Answer from the drawing. Dimensions are ordinates in mm from the lowest x, y and z of the part. A direction names the side the tool comes from. Coordinates: 2 decimals unless noted, no trailing zeros. Loops run counter-clockwise (first coordinate to the right, second up) from the corner with the lowest first, then second, coordinate; pieces in that order, holes last.
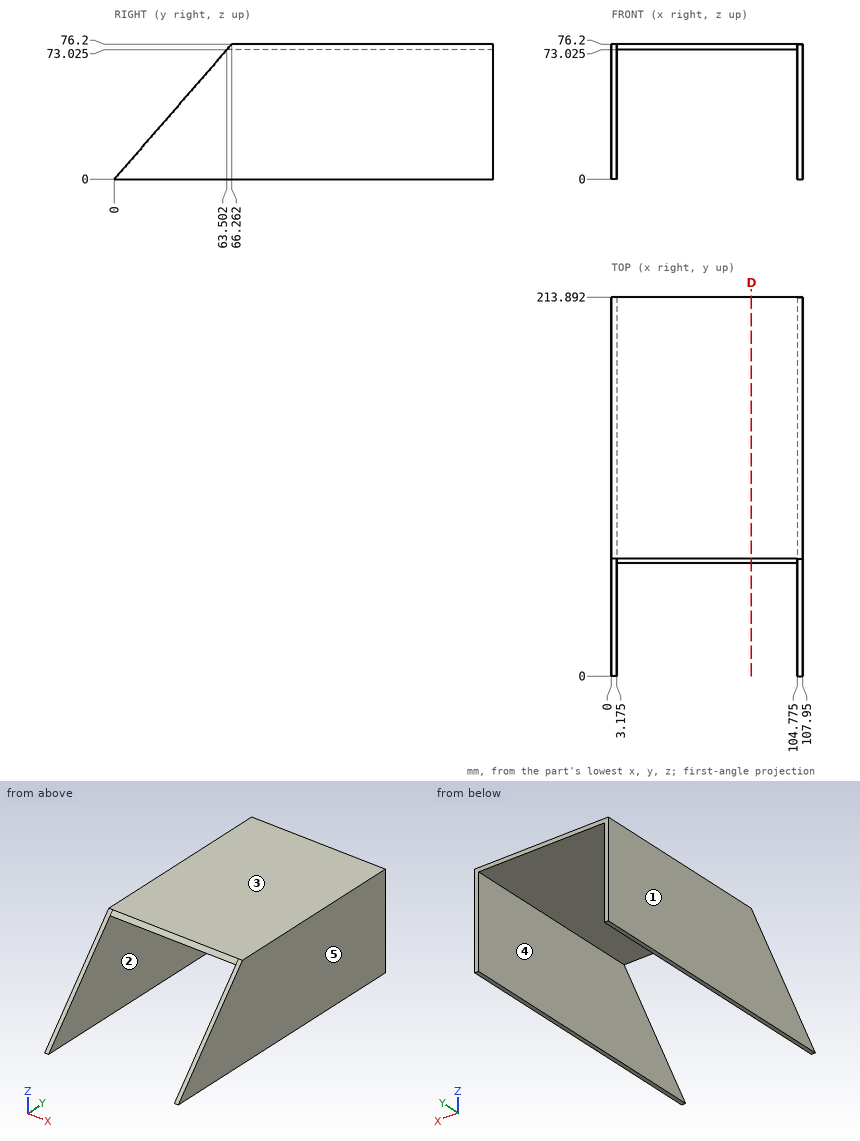
Item 1: Determine the mould class of the marked faces 1, 2 and 3 for opening direction X: released by +X, released by -X, zero draft, split by the parting line, or undercut.
Numbers:
face 1: released by -X
face 2: undercut
face 3: zero draft
Item 2: A cutting plane is placed at D-D on x = 79. Determine the outline of the cut face in (y, z) (1 decimal).
Numbers:
outline: (63.5, 73) - (213.9, 73) - (213.9, 76.2) - (66.3, 76.2) - close
Item 3: Given pin 1 (4 mm diameter, centred on y = 160, z = 60.5, fed in from -X); pin 2 (3 mm diameter, centred on x = 72.5, y = 154.5, fed in from -Z) (3 decimals), each flat-ended and moving along its own axis, determine where each tip first touches the part or whether it passes through.
Numbers:
pin 1: stops at x = 0
pin 2: stops at z = 73.025
Item 4: Which of the six approach directions +Z, -Z, +X, -X, +Y, -Y give full straight-line access (tool end or side, diameter ignored) to the marked faces 4 and 5?
Numbers:
face 4: -Z, +Y, -Y
face 5: +Z, -Z, +X, +Y, -Y
Item 5: Find the intervals of material crossed by line 1 along Z through (x, y) = (56.5, 181) (1 decimal), in increasing order.
Numbers:
line 1: z = 73 to 76.2
